Check sheet for the modelled part. Datum: model origin and axes. Units: mm. Give positions to 0.01 mm unless a question says otherwise; leave off trailing zeros. Loops run counter-clockwise (first coordinate to the right, second up) from the corner with the lowest first, then second, coordinate; pieces in that order, holes last. Notation, with made-up numbers: (-2.75, -7.75) -> (26.25, -7.75) arc R17 ccw to (26.25, 23.25) -> close; hole circle Ø10 at (25, 12). An arc over 180 degrees is marked (long way). Answer as CSV lines item,"result". Start each with the question number.
(1) Material ranges on line 1 (Y direction, x = 0, z = 1.2); line 2 (Y direction, x = -7, z = 1.35); line 3 (X direction, y = 4, z = 1.1), recorded low to high. Write a range as from..to.
(2) Section check A-A on x = 0. Enter the section's corners in (y, z).
(3) Gauge pin test, flat end, axial feed: pin 1 Ø2 at (x, y) = (0, 123.19) entering from +Z. Record the tip position at first contact, or that the pin passes through.
(4) Section check C-C on x = -7. Enter the section's corners in (y, z).
(5) Section check B-B on z = 0.65. State how many separate pieces and enclosed holes the cut face has, plus the area to 3 significant figures.
from build123d import *

# Parameters (mm, degrees)
ESBO_O1_R                = 1.35
ESBO_O1_R_2              = 5.05
RESSALTO_EXTRUS_O1_DEPTH = 1.8
FILETE1_R                = 3
FILETE2_R                = 3


with BuildPart() as part:
    # Esboço1 → Ressalto-extrusão1 (new body)
    with BuildSketch(Plane.XY):
        with BuildLine():
            Line((-12.596174938, 0), (-12.596174938, 145.832394841))
            Line((-12.596174938, 145.832394841), (12.596174938, 145.832394841))
            Line((12.596174938, 145.832394841), (12.596174938, 0))
            ThreePointArc((12.596174938, 0), (0, -12.596174938), (-12.596174938, 0))
        make_face()
        with Locations((7, 41.089981595)):
            Circle(ESBO_O1_R, mode=Mode.SUBTRACT)
        with Locations((7, 69.089981595)):
            Circle(ESBO_O1_R, mode=Mode.SUBTRACT)
        with Locations(Location((-7, 41.089981595, 0), (0, 0, 180))):
            Circle(ESBO_O1_R, mode=Mode.SUBTRACT)
        with Locations(Location((-7, 69.089981595, 0), (0, 0, 180))):
            Circle(ESBO_O1_R, mode=Mode.SUBTRACT)
        with Locations((7, 130.185826181)):
            Circle(ESBO_O1_R, mode=Mode.SUBTRACT)
        with Locations((0, 137.185826181)):
            Circle(ESBO_O1_R, mode=Mode.SUBTRACT)
        with Locations(Location((-7, 130.185826181, 0), (0, 0, 180))):
            Circle(ESBO_O1_R, mode=Mode.SUBTRACT)
        with Locations(Location((0, 123.185826181, 0), (0, 0, 180))):
            Circle(ESBO_O1_R, mode=Mode.SUBTRACT)
        Circle(ESBO_O1_R_2, mode=Mode.SUBTRACT)
    extrude(amount=RESSALTO_EXTRUS_O1_DEPTH)

    # Filete1
    filete1_edges = [part.edges().sort_by_distance(p)[0] for p in [
        (-12.596174938, 145.832394841, 0.9),
    ]]
    fillet(filete1_edges, radius=FILETE1_R)

    # Filete2
    filete2_edges = [part.edges().sort_by_distance(p)[0] for p in [
        (12.596174938, 145.832394841, 0.9),
    ]]
    fillet(filete2_edges, radius=FILETE2_R)


solid = part.part
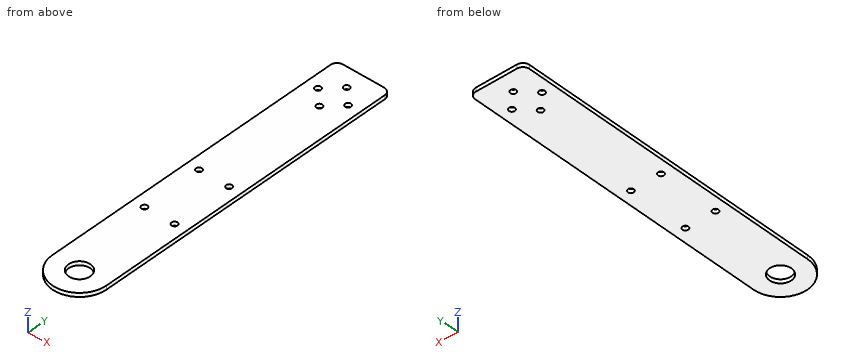
Working result:
1,line 1,"y = -12.6..-5.05, 5.05..121.84, 124.54..135.84, 138.54..145.83"
1,line 2,"y = -10.47..39.74, 42.44..67.74, 70.44..128.84, 131.54..145.83"
1,line 3,"x = -12.6..-3.08, 3.08..12.6"
2,outline,"(-12.6, 0) -> (-5.05, 0) -> (-5.05, 1.8) -> (-12.6, 1.8) -> close; (5.05, 0) -> (121.84, 0) -> (121.84, 1.8) -> (5.05, 1.8) -> close; (124.54, 0) -> (135.84, 0) -> (135.84, 1.8) -> (124.54, 1.8) -> close; (138.54, 0) -> (145.83, 0) -> (145.83, 1.8) -> (138.54, 1.8) -> close"
3,pin 1,"passes through"
4,outline,"(-10.47, 0) -> (39.74, 0) -> (39.74, 1.8) -> (-10.47, 1.8) -> close; (42.44, 0) -> (67.74, 0) -> (67.74, 1.8) -> (42.44, 1.8) -> close; (70.44, 0) -> (128.84, 0) -> (128.84, 1.8) -> (70.44, 1.8) -> close; (131.54, 0) -> (145.83, 0) -> (145.83, 1.8) -> (131.54, 1.8) -> close"
5,separate pieces,"1"
5,enclosed holes,"9"
5,area,"3,790 mm^2"
